Source: CAD feature listing. Evaluate the final solid. Frame: model axes, mm. A direction names the side the tool comes from. Round coordinates to 2 decimals unless told otherwise and drop trailing zeros. Order: outer loops, then holes, each group sorted by start corner. A loop starts at its lowest first (then second) coordinate and runs counter-clockwise, first axis right, second up. Notation, with made-up numbers: (76, -5.5) - (94, -5.5) arc R23 cw to (94, 25.5) - close; hole circle Ø1 at (59.5, 65). An arc over 180 degrees is marked (long way). Put each result on its own line as item: value. Start each with the question number.
1) Mould query, pull axis X, two halves, no side actions, for faces 4 (the face through (-17, -5, 0)), 5 (the face through (-16.155, -5, 10)), 6 (the face through (-20.424, -5, 57)), 7 (the face through (-33.424, -5, 47)). Classes: +X half, -X half, draft (parallel to the pull), parting line (faces both ways), or undercut.
2) Access query for faces 1 (the face through (-24.424, -5, 57)), 2 (the face through (-23, 19.75, 36)), 3 (the face through (-19, -5, 20)). Directions: +Z, -Z, +X, -X, +Y, -Y. A direction counts if a zero-diameter tool reaches every point of the face in a straight line with its end or side. Return the directions, or none.
3) Line query: probe 1 along X at (y, z) = (-21, 78.5); probe 2 along X at (y, z) = (36.5, 17.5); probe 3 along Y at (x, z) = (-23.5, 29). Output: solid intervals per line, ascending. Write a range as [from, to].
4) Contact query for flat-ended pins moving along their axis: P1, Ø3, axis at x = -6.5, y = -45.5, coming from the -Z side; P2, Ø2, axis at y = -29, z = 10.5, coming from the +X side; P3, Ø19, axis at x = -22, z = 43, coming from the -Y side (3 decimals); P4, Ø2, axis at y = 19, z = 14.5, coming from the +X side. Output: stop coordinate, or through.
5) Section B-B on y = -3.5. Output: boundary loops of the cut face in (x, z), then the cut area to 3 significant figures.
6) Section C-C on x = 33. Output: boundary loops of the cut face in (y, z), then the cut area to 3 significant figures.
7) Section D-D on z = 16. Output: boundary loops of the cut face in (x, y), then the cut area to 3 significant figures.
8) Section A-A on z = 36. Output: boundary loops of the cut face in (x, y), then the cut area to 3 significant figures.
```python
from build123d import *

# Parameters (mm, degrees)
SKETCH_1_R      = 57.5
SKETCH_1_R_2    = 55
SKETCH_1_W      = 17.269051877
SKETCH_1_H      = 49.42521744
EXTRUDE_1_DEPTH = 20
SKETCH_2_W      = 4
SKETCH_2_H      = 49.42521744
EXTRUDE_2_DEPTH = 75


with BuildPart() as part:
    # 草圖1 → 填料-伸長1 (new body)
    # profile 1 of 2: a face of its own
    with BuildSketch(Plane.XY):
        with Locations((36.644946032, -4.863123804)):
            Circle(SKETCH_1_R)
        with Locations((36.644946032, -4.863123804)):
            Circle(SKETCH_1_R_2, mode=Mode.SUBTRACT)
    # profile 2 of 2: a face of its own
    with BuildSketch(Plane.XY):
        with Locations((-24.789209782, -4.962371229)):
            Rectangle(SKETCH_1_W, SKETCH_1_H)
    extrude(amount=EXTRUDE_1_DEPTH)

    # 草圖2 → 填料-伸長2 (add)
    with BuildSketch(Plane.XY.offset(20)):
        with Locations((-31.42373572, -4.962371229)):
            Rectangle(SKETCH_2_W, SKETCH_2_H)
        with Locations((-22.42373572, -4.962371229)):
            Rectangle(SKETCH_2_W, SKETCH_2_H)
    extrude(amount=EXTRUDE_2_DEPTH)


solid = part.part
```
Answer sheet:
1. face 4: draft
1. face 5: undercut
1. face 6: +X half
1. face 7: -X half
2. face 1: +Z, +Y, -Y
2. face 2: +Z, -Z, -X, +Y
2. face 3: +Z, +X, +Y, -Y
3. probe 1: [-33.42, -29.42], [-24.42, -20.42]
3. probe 2: [-3.3, 0.39], [72.9, 76.59]
3. probe 3: [-29.67, 19.75]
4. P1: through
4. P2: x = 89.28
4. P3: y = -29.675
4. P4: x = 89.4
5. outline: (-33.42, 0) - (-16.15, 0) - (-16.15, 20) - (-20.42, 20) - (-20.42, 95) - (-24.42, 95) - (-24.42, 20) - (-29.42, 20) - (-29.42, 95) - (-33.42, 95) - close; (91.63, 0) - (94.13, 0) - (94.13, 20) - (91.63, 20) - close
5. area: 995 mm^2
6. outline: (-62.25, 0) - (-59.74, 0) - (-59.74, 20) - (-62.25, 20) - close; (50.02, 0) - (52.52, 0) - (52.52, 20) - (50.02, 20) - close
6. area: 100 mm^2
7. outline: (-33.42, -29.67) - (-16.15, -29.67) - (-16.15, -27.63) arc R57.5 ccw (long way) to (-16.15, 17.91) - (-16.15, 19.75) - (-33.42, 19.75) - close; hole (-16.15, -20.26) arc R55 ccw (long way) to (-16.15, 10.54) - close
7. area: 1,640 mm^2
8. outline: (-33.42, -29.67) - (-29.42, -29.67) - (-29.42, 19.75) - (-33.42, 19.75) - close; (-24.42, -29.67) - (-20.42, -29.67) - (-20.42, 19.75) - (-24.42, 19.75) - close
8. area: 395 mm^2
